Can you work these out from the model? Positions are in its coordinate system, mm. Round coordinates to 2 decimals unless told otherwise and drop trailing zeros. Loops run counter-clockwise (first coordinate to the right, second up) from the corner with the lowest first, then second, coordinate; pieces in that order, holes last.
(1) Thinking about a two-plate mould opening in X: for faces 1 (the face through (31, 21.07, 2.03)), 2 (the face through (-26.21, -16.32, 1.97)), 3 (the face through (0, 0, 4)), which applies, released by +X, released by -X, zero draft, split by the parting line, or undercut?
(2) I want a section at A-A on z = 0.6. Write out the boundary of the cut face in (x, y).
(3) If I drill on line 1 along Y through (x, z) = (-27.5, 2.6); line 2 along Y through (x, z) = (-26, 0.7); line 3 along X through (y, z) = (-19, 1.8), over which ranges is the centre line in solid material (lowest first)?
from build123d import *

# Parameters (mm, degrees)
SKETCH_1_W              = 65
SKETCH_1_H              = 45
EXTRUDE_1_DEPTH         = 4
HOLE_WIZARD_3_5_3_5_1_D = 3.5
FILLET_1_R              = 5


with BuildPart() as part:
    # 草图1 → 凸台-拉伸1 (new body)
    with BuildSketch(Plane.XY):
        Rectangle(SKETCH_1_W, SKETCH_1_H)
    extrude(amount=EXTRUDE_1_DEPTH)

    # Ø3.5 (3.5) 直径孔1 (through all)
    with Locations(Plane.XY.offset(4)):
        with Locations((-27.5, 17.5), (-27.5, -17.5), (27.5, 17.5), (27.5, -17.5)):
            Hole(HOLE_WIZARD_3_5_3_5_1_D / 2)

    # 圆角1
    fillet_1_edges = [part.edges().sort_by_distance(p)[0] for p in [
        (32.5, -22.5, 2),
        (-32.5, -22.5, 2),
        (-32.5, 22.5, 2),
        (32.5, 22.5, 2),
    ]]
    fillet(fillet_1_edges, radius=FILLET_1_R)


solid = part.part
Filled sheet:
1. face 1: released by +X
1. face 2: undercut
1. face 3: zero draft
2. outline: (-32.5, -17.5) arc R5 ccw to (-27.5, -22.5) - (27.5, -22.5) arc R5 ccw to (32.5, -17.5) - (32.5, 17.5) arc R5 ccw to (27.5, 22.5) - (-27.5, 22.5) arc R5 ccw to (-32.5, 17.5) - close; hole circle Ø3.5 at (-27.5, -17.5); hole circle Ø3.5 at (-27.5, 17.5); hole circle Ø3.5 at (27.5, -17.5); hole circle Ø3.5 at (27.5, 17.5)
3. line 1: y = -22.5 to -19.25, -15.75 to 15.75, 19.25 to 22.5
3. line 2: y = -22.5 to -18.4, -16.6 to 16.6, 18.4 to 22.5
3. line 3: x = -32.27 to -28.4, -26.6 to 26.6, 28.4 to 32.27
